Source: CAD feature listing. Evaluate the final solid. Frame: model axes, mm. A direction names the side the tool comes from. Give positions to 0.01 mm unless a question says otherwise; leave off trailing zeros. Write each loop counter-clockwise with the first axis right and the second up, starting at its lowest first coordinate (ties: lowest second). Pieces come first, ordered by that corner, then holes.
```python
from build123d import *

# Parameters (mm, degrees)
SKETCH1_W           = 304.8
SKETCH1_H           = 304.8
BOSS_EXTRUDE1_DEPTH = 6.35
SKETCH2_R           = 25.4
CUT_EXTRUDE2_DEPTH  = 432.099063441


with BuildPart() as part:
    # Sketch1 → Boss-Extrude1 (new body)
    with BuildSketch(Plane(origin=(0, 0, 0), x_dir=(1, 0, 0), z_dir=(0, 1, 0))):
        with Locations((152.4, 152.4)):
            Rectangle(SKETCH1_W, SKETCH1_H)
    extrude(amount=BOSS_EXTRUDE1_DEPTH)

    # Sketch2 → Cut-Extrude2 (cut, through all)
    with BuildSketch(Plane(origin=(0, 6.35, 0), x_dir=(1, 0, 0), z_dir=(0, 1, 0))):
        with Locations(Location((40.378551944, 126.297217899, 0), (0, 0, 270))):
            Circle(SKETCH2_R)
        with Locations(Location((93.964492013, 129.211934304, 0), (0, 0, 270))):
            Circle(SKETCH2_R)
        with Locations(Location((130.510551558, 167.551665483, 0), (0, 0, 270))):
            Circle(SKETCH2_R)
        with Locations(Location((171.52597858, 133.696113389, 0), (0, 0, 270))):
            Circle(SKETCH2_R)
        with BuildLine():
            Line((12.7, 289.56), (12.7, 247.432102448))
            ThreePointArc((12.7, 247.432102448), (14.267984082, 245.085448436), (17.036051224, 245.636051224))
            Line((17.036051224, 245.636051224), (59.163948776, 287.763948776))
            ThreePointArc((59.163948776, 287.763948776), (59.714551564, 290.532015918), (57.367897552, 292.1))
            Line((57.367897552, 292.1), (15.24, 292.1))
            ThreePointArc((15.24, 292.1), (13.443948776, 291.356051224), (12.7, 289.56))
        make_face()
        with BuildLine():
            Line((67.836051224, 245.636051224), (109.963948776, 287.763948776))
            ThreePointArc((109.963948776, 287.763948776), (110.514551564, 290.532015918), (108.167897552, 292.1))
            Line((108.167897552, 292.1), (66.04, 292.1))
            ThreePointArc((66.04, 292.1), (64.243948776, 291.356051224), (63.5, 289.56))
            Line((63.5, 289.56), (63.5, 247.432102448))
            ThreePointArc((63.5, 247.432102448), (65.067984082, 245.085448436), (67.836051224, 245.636051224))
        make_face()
        with BuildLine():
            Line((118.636051224, 245.636051224), (160.763948776, 287.763948776))
            ThreePointArc((160.763948776, 287.763948776), (161.314551564, 290.532015918), (158.967897552, 292.1))
            Line((158.967897552, 292.1), (116.84, 292.1))
            ThreePointArc((116.84, 292.1), (115.043948776, 291.356051224), (114.3, 289.56))
            Line((114.3, 289.56), (114.3, 247.432102448))
            ThreePointArc((114.3, 247.432102448), (115.867984082, 245.085448436), (118.636051224, 245.636051224))
        make_face()
        with BuildLine():
            Line((169.436051224, 245.636051224), (211.563948776, 287.763948776))
            ThreePointArc((211.563948776, 287.763948776), (212.114551564, 290.532015918), (209.767897552, 292.1))
            Line((209.767897552, 292.1), (167.64, 292.1))
            ThreePointArc((167.64, 292.1), (165.843948776, 291.356051224), (165.1, 289.56))
            Line((165.1, 289.56), (165.1, 247.432102448))
            ThreePointArc((165.1, 247.432102448), (166.667984082, 245.085448436), (169.436051224, 245.636051224))
        make_face()
        with BuildLine():
            Line((220.236051224, 245.636051224), (262.363948776, 287.763948776))
            ThreePointArc((262.363948776, 287.763948776), (262.914551564, 290.532015918), (260.567897552, 292.1))
            Line((260.567897552, 292.1), (218.44, 292.1))
            ThreePointArc((218.44, 292.1), (216.643948776, 291.356051224), (215.9, 289.56))
            Line((215.9, 289.56), (215.9, 247.432102448))
            ThreePointArc((215.9, 247.432102448), (217.467984082, 245.085448436), (220.236051224, 245.636051224))
        make_face()
        with BuildLine():
            Line((67.836051224, 194.836051224), (109.963948776, 236.963948776))
            ThreePointArc((109.963948776, 236.963948776), (110.514551564, 239.732015918), (108.167897552, 241.3))
            Line((108.167897552, 241.3), (66.04, 241.3))
            ThreePointArc((66.04, 241.3), (64.243948776, 240.556051224), (63.5, 238.76))
            Line((63.5, 238.76), (63.5, 196.632102448))
            ThreePointArc((63.5, 196.632102448), (65.067984082, 194.285448436), (67.836051224, 194.836051224))
        make_face()
        with BuildLine():
            Line((118.636051224, 194.836051224), (160.763948776, 236.963948776))
            ThreePointArc((160.763948776, 236.963948776), (161.314551564, 239.732015918), (158.967897552, 241.3))
            Line((158.967897552, 241.3), (116.84, 241.3))
            ThreePointArc((116.84, 241.3), (115.043948776, 240.556051224), (114.3, 238.76))
            Line((114.3, 238.76), (114.3, 196.632102448))
            ThreePointArc((114.3, 196.632102448), (115.867984082, 194.285448436), (118.636051224, 194.836051224))
        make_face()
        with BuildLine():
            Line((169.436051224, 194.836051224), (211.563948776, 236.963948776))
            ThreePointArc((211.563948776, 236.963948776), (212.114551564, 239.732015918), (209.767897552, 241.3))
            Line((209.767897552, 241.3), (167.64, 241.3))
            ThreePointArc((167.64, 241.3), (165.843948776, 240.556051224), (165.1, 238.76))
            Line((165.1, 238.76), (165.1, 196.632102448))
            ThreePointArc((165.1, 196.632102448), (166.667984082, 194.285448436), (169.436051224, 194.836051224))
        make_face()
        with BuildLine():
            Line((220.236051224, 194.836051224), (262.363948776, 236.963948776))
            ThreePointArc((262.363948776, 236.963948776), (262.914551564, 239.732015918), (260.567897552, 241.3))
            Line((260.567897552, 241.3), (218.44, 241.3))
            ThreePointArc((218.44, 241.3), (216.643948776, 240.556051224), (215.9, 238.76))
            Line((215.9, 238.76), (215.9, 196.632102448))
            ThreePointArc((215.9, 196.632102448), (217.467984082, 194.285448436), (220.236051224, 194.836051224))
        make_face()
        with BuildLine():
            Line((17.036051224, 194.836051224), (59.163948776, 236.963948776))
            ThreePointArc((59.163948776, 236.963948776), (59.714551564, 239.732015918), (57.367897552, 241.3))
            Line((57.367897552, 241.3), (15.24, 241.3))
            ThreePointArc((15.24, 241.3), (13.443948776, 240.556051224), (12.7, 238.76))
            Line((12.7, 238.76), (12.7, 196.632102448))
            ThreePointArc((12.7, 196.632102448), (14.267984082, 194.285448436), (17.036051224, 194.836051224))
        make_face()
        with BuildLine():
            Line((17.036051224, 144.036051224), (59.163948776, 186.163948776))
            ThreePointArc((59.163948776, 186.163948776), (59.714551564, 188.932015918), (57.367897552, 190.5))
            Line((57.367897552, 190.5), (15.24, 190.5))
            ThreePointArc((15.24, 190.5), (13.443948776, 189.756051224), (12.7, 187.96))
            Line((12.7, 187.96), (12.7, 145.832102448))
            ThreePointArc((12.7, 145.832102448), (14.267984082, 143.485448436), (17.036051224, 144.036051224))
        make_face()
        with BuildLine():
            Line((67.836051224, 144.036051224), (109.963948776, 186.163948776))
            ThreePointArc((109.963948776, 186.163948776), (110.514551564, 188.932015918), (108.167897552, 190.5))
            Line((108.167897552, 190.5), (66.04, 190.5))
            ThreePointArc((66.04, 190.5), (64.243948776, 189.756051224), (63.5, 187.96))
            Line((63.5, 187.96), (63.5, 145.832102448))
            ThreePointArc((63.5, 145.832102448), (65.067984082, 143.485448436), (67.836051224, 144.036051224))
        make_face()
        with BuildLine():
            Line((12.7, 15.24), (12.7, 103.540387337))
            ThreePointArc((12.7, 103.540387337), (14.656427582, 106.01243977), (17.511845065, 104.67630987))
            Line((17.511845065, 104.67630987), (61.662038734, 16.375922533))
            ThreePointArc((61.662038734, 16.375922533), (61.550846722, 13.904642975), (59.390193669, 12.7))
            Line((59.390193669, 12.7), (15.24, 12.7))
            ThreePointArc((15.24, 12.7), (13.443948776, 13.443948776), (12.7, 15.24))
        make_face()
        with BuildLine():
            Line((68.311845065, 104.67630987), (112.462038734, 16.375922533))
            ThreePointArc((112.462038734, 16.375922533), (112.350846722, 13.904642975), (110.190193669, 12.7))
            Line((110.190193669, 12.7), (66.04, 12.7))
            ThreePointArc((66.04, 12.7), (64.243948776, 13.443948776), (63.5, 15.24))
            Line((63.5, 15.24), (63.5, 103.540387337))
            ThreePointArc((63.5, 103.540387337), (65.456427582, 106.01243977), (68.311845065, 104.67630987))
        make_face()
        with BuildLine():
            Line((119.111845065, 104.67630987), (163.262038734, 16.375922533))
            ThreePointArc((163.262038734, 16.375922533), (163.150846722, 13.904642975), (160.990193669, 12.7))
            Line((160.990193669, 12.7), (116.84, 12.7))
            ThreePointArc((116.84, 12.7), (115.043948776, 13.443948776), (114.3, 15.24))
            Line((114.3, 15.24), (114.3, 103.540387337))
            ThreePointArc((114.3, 103.540387337), (116.256427582, 106.01243977), (119.111845065, 104.67630987))
        make_face()
        with BuildLine():
            Line((169.911845065, 104.67630987), (214.062038734, 16.375922533))
            ThreePointArc((214.062038734, 16.375922533), (213.950846722, 13.904642975), (211.790193669, 12.7))
            Line((211.790193669, 12.7), (167.64, 12.7))
            ThreePointArc((167.64, 12.7), (165.843948776, 13.443948776), (165.1, 15.24))
            Line((165.1, 15.24), (165.1, 103.540387337))
            ThreePointArc((165.1, 103.540387337), (167.056427582, 106.01243977), (169.911845065, 104.67630987))
        make_face()
        with BuildLine():
            Line((220.711845065, 104.67630987), (264.862038734, 16.375922533))
            ThreePointArc((264.862038734, 16.375922533), (264.750846722, 13.904642975), (262.590193669, 12.7))
            Line((262.590193669, 12.7), (218.44, 12.7))
            ThreePointArc((218.44, 12.7), (216.643948776, 13.443948776), (215.9, 15.24))
            Line((215.9, 15.24), (215.9, 103.540387337))
            ThreePointArc((215.9, 103.540387337), (217.856427582, 106.01243977), (220.711845065, 104.67630987))
        make_face()
        with BuildLine():
            Line((277.552172751, 15.24), (233.401979083, 103.540387337))
            ThreePointArc((233.401979083, 103.540387337), (233.513171095, 106.011666895), (235.673824148, 107.21630987))
            Line((235.673824148, 107.21630987), (279.824017817, 107.21630987))
            ThreePointArc((279.824017817, 107.21630987), (281.620069041, 106.472361094), (282.364017817, 104.67630987))
            Line((282.364017817, 104.67630987), (282.364017817, 16.375922533))
            ThreePointArc((282.364017817, 16.375922533), (280.407590235, 13.903870099), (277.552172751, 15.24))
        make_face()
        with BuildLine():
            Line((291.693726792, 146.554658473), (203.393339455, 102.404464805))
            ThreePointArc((203.393339455, 102.404464805), (200.922059898, 102.515656817), (199.717416922, 104.67630987))
            Line((199.717416922, 104.67630987), (199.717416922, 148.826503538))
            ThreePointArc((199.717416922, 148.826503538), (200.461365698, 150.622554763), (202.257416922, 151.366503538))
            Line((202.257416922, 151.366503538), (290.55780426, 151.366503538))
            ThreePointArc((290.55780426, 151.366503538), (293.029856693, 149.410075956), (291.693726792, 146.554658473))
        make_face()
        with BuildLine():
            Line((183.6711366, 168.254047869), (271.971523937, 212.404241537))
            ThreePointArc((271.971523937, 212.404241537), (274.442803495, 212.293049525), (275.64744647, 210.132396472))
            Line((275.64744647, 210.132396472), (275.64744647, 165.982202803))
            ThreePointArc((275.64744647, 165.982202803), (274.903497694, 164.186151579), (273.10744647, 163.442202803))
            Line((273.10744647, 163.442202803), (184.807059133, 163.442202803))
            ThreePointArc((184.807059133, 163.442202803), (182.335006699, 165.398630385), (183.6711366, 168.254047869))
        make_face()
    extrude(amount=-CUT_EXTRUDE2_DEPTH, mode=Mode.SUBTRACT)


solid = part.part
```
1. Section query A-A (z = -268.5). Return loops of the section in (x, y).
2. Section query B-B (x = 247). Return loops of the section in (y, z).
3. Section query C-C (z = -114). Return loops of the section in (x, y), plus the area to 3 significant figures.
4. Section query D-D (z = -27). Return loops of the section in (x, y), plus the area to 3 significant figures.
5. Line query: probe 1 along Z at (x, y) = (181.5, 4.5); probe 2 along X at (y, z) = (4, -175.5); probe 3 along X at (y, z) = (1.5, -183). Output: solid intervals per line, ascending.
6. Access query for faces 3 (the flat face through (38, 3, -165)), 4 (the flat face through (184, 0, -188)). Directions: +Z, -Z, +X, -X, +Y, -Y. A direction counts if a zero-diameter tool reaches every point of the face in a straight line with its end or side. Return the directions, or none.
7. Pin query (flat end, axial travel): P1, Ø3, axis at x = 196.5, y = 3, coming from the +Z side. Return the tip coordinate at first contact, or that it passes through.
8. Pull-direction query (X, two-part tool) for faces 1 (the cylindrical face through (196.71, 3.22, -137)), 2 (the flat face through (184, 6.35, -188)); classes: pulls with the +X half, pulls with the -X half, needs draft (parallel to the pull), parting line crosses it, or undercut.
The answers:
1. outline: (0, 0) - (12.7, 0) - (12.7, 6.35) - (0, 6.35) - close; (39.9, 0) - (63.5, 0) - (63.5, 6.35) - (39.9, 6.35) - close; (90.7, 0) - (114.3, 0) - (114.3, 6.35) - (90.7, 6.35) - close; (141.5, 0) - (165.1, 0) - (165.1, 6.35) - (141.5, 6.35) - close; (192.3, 0) - (215.9, 0) - (215.9, 6.35) - (192.3, 6.35) - close; (243.1, 0) - (304.8, 0) - (304.8, 6.35) - (243.1, 6.35) - close
2. outline: (0, -304.8) - (6.35, -304.8) - (6.35, -292.1) - (0, -292.1) - close; (0, -272.4) - (6.35, -272.4) - (6.35, -241.3) - (0, -241.3) - close; (0, -221.6) - (6.35, -221.6) - (6.35, -199.92) - (0, -199.92) - close; (0, -163.44) - (6.35, -163.44) - (6.35, -151.37) - (0, -151.37) - close; (0, -124.21) - (6.35, -124.21) - (6.35, -107.22) - (0, -107.22) - close; (0, -76.34) - (6.35, -76.34) - (6.35, -52.1) - (0, -52.1) - close; (0, -12.7) - (6.35, -12.7) - (6.35, 0) - (0, 0) - close
3. outline: (0, 0) - (18.15, 0) - (18.15, 6.35) - (0, 6.35) - close; (62.6, 0) - (73.62, 0) - (73.62, 6.35) - (62.6, 6.35) - close; (114.31, 0) - (155.49, 0) - (155.49, 6.35) - (114.31, 6.35) - close; (187.56, 0) - (199.72, 0) - (199.72, 6.35) - (187.56, 6.35) - close; (226.58, 0) - (304.8, 0) - (304.8, 6.35) - (226.58, 6.35) - close
3. area: 1,020 mm2
4. outline: (0, 0) - (12.7, 0) - (12.7, 6.35) - (0, 6.35) - close; (56.35, 0) - (63.5, 0) - (63.5, 6.35) - (56.35, 6.35) - close; (107.15, 0) - (114.3, 0) - (114.3, 6.35) - (107.15, 6.35) - close; (157.95, 0) - (165.1, 0) - (165.1, 6.35) - (157.95, 6.35) - close; (208.75, 0) - (215.9, 0) - (215.9, 6.35) - (208.75, 6.35) - close; (259.55, 0) - (271.67, 0) - (271.67, 6.35) - (259.55, 6.35) - close; (282.36, 0) - (304.8, 0) - (304.8, 6.35) - (282.36, 6.35) - close
4. area: 482 mm2
5. probe 1: z = -304.8 to -292.1, -257.7 to -241.3, -206.9 to -157.06, -110.34 to -81.5, -12.7 to 0
5. probe 2: x = 0 to 12.7, 48.5 to 63.5, 99.3 to 106.39, 154.63 to 198.16, 275.65 to 304.8
5. probe 3: x = 0 to 12.7, 56 to 63.5, 106.8 to 110.35, 150.67 to 213.16, 275.65 to 304.8
6. face 3: +Y, -Y
6. face 4: +Z, -Z, +X, -X, -Y
7. P1: stops at z = 0
8. face 1: undercut
8. face 2: needs draft
